```python
from build123d import *

# Parameters (mm, degrees)
SKETCH1_R           = 2.25
SKETCH1_R_2         = 1.5
BOSS_EXTRUDE1_DEPTH = 3


with BuildPart() as part:
    # Sketch1 → Boss-Extrude1 (new body)
    with BuildSketch(Plane.XY):
        with BuildLine():
            Line((-43.5, -20.5), (-47.6, -20.5))
            ThreePointArc((-47.6, -20.5), (-49.014213562, -19.914213562), (-49.6, -18.5))
            Line((-49.6, -18.5), (-49.6, 5))
            ThreePointArc((-49.6, 5), (-49.468344718, 5.71364418), (-49.090711985, 6.333333333))
            ThreePointArc((-49.090711985, 6.333333333), (-48.836067978, 7), (-49.090711985, 7.666666667))
            ThreePointArc((-49.090711985, 7.666666667), (-49.468344718, 8.28635582), (-49.6, 9))
            Line((-49.6, 9), (-49.6, 35))
            ThreePointArc((-49.6, 35), (-49.468344718, 35.71364418), (-49.090711985, 36.333333333))
            ThreePointArc((-49.090711985, 36.333333333), (-48.836067978, 37), (-49.090711985, 37.666666667))
            ThreePointArc((-49.090711985, 37.666666667), (-49.468344718, 38.28635582), (-49.6, 39))
            Line((-49.6, 39), (-49.6, 62.5))
            ThreePointArc((-49.6, 62.5), (-49.014213562, 63.914213562), (-47.6, 64.5))
            Line((-47.6, 64.5), (6.1, 64.5))
            ThreePointArc((6.1, 64.5), (7.514213562, 63.914213562), (8.1, 62.5))
            Line((8.1, 62.5), (8.1, 39))
            ThreePointArc((8.1, 39), (7.968344718, 38.28635582), (7.590711985, 37.666666667))
            ThreePointArc((7.590711985, 37.666666667), (7.336067978, 37), (7.590711985, 36.333333333))
            ThreePointArc((7.590711985, 36.333333333), (7.968344718, 35.71364418), (8.1, 35))
            Line((8.1, 35), (8.1, 9))
            ThreePointArc((8.1, 9), (7.968344718, 8.28635582), (7.590711985, 7.666666667))
            ThreePointArc((7.590711985, 7.666666667), (7.336067978, 7), (7.590711985, 6.333333333))
            ThreePointArc((7.590711985, 6.333333333), (7.968344718, 5.71364418), (8.1, 5))
            Line((8.1, 5), (8.1, -18.5))
            ThreePointArc((8.1, -18.5), (7.514213562, -19.914213562), (6.1, -20.5))
            Line((6.1, -20.5), (2, -20.5))
            ThreePointArc((2, -20.5), (0.585786438, -19.914213562), (0, -18.5))
            Line((0, -18.5), (0, 0))
            Line((0, 0), (-41.5, 0))
            Line((-41.5, 0), (-41.5, -18.5))
            ThreePointArc((-41.5, -18.5), (-42.085786438, -19.914213562), (-43.5, -20.5))
        make_face()
        with Locations((-45.55, -5.5)):
            Circle(SKETCH1_R, mode=Mode.SUBTRACT)
        with Locations((-45.55, -15)):
            Circle(SKETCH1_R, mode=Mode.SUBTRACT)
        with Locations((4.05, -5.5)):
            Circle(SKETCH1_R, mode=Mode.SUBTRACT)
        with Locations((4.05, -15)):
            Circle(SKETCH1_R, mode=Mode.SUBTRACT)
        with Locations((-30.55, 17)):
            Circle(SKETCH1_R, mode=Mode.SUBTRACT)
        with Locations((-30.55, 27)):
            Circle(SKETCH1_R, mode=Mode.SUBTRACT)
        with Locations((-10.14, 54.25)):
            Circle(SKETCH1_R_2, mode=Mode.SUBTRACT)
    extrude(amount=BOSS_EXTRUDE1_DEPTH)


solid = part.part
```
Can you work these out from the model? Positions are in its coordinate system, mm. A direction names the side the tool comes from. Round coordinates to 2 decimals unless told otherwise and drop trailing zeros. Loops run counter-clockwise (first coordinate to the right, second up) from the corner with the lowest first, then second, coordinate; pieces in that order, holes last.
Item 1: Will these pins go through, and if not, where does the flat tip stop? pin 1 Ø5 at (x, y) = (-30.55, 17) entering from -Z; pin 2 Ø0.9 at (x, z) = (-16.5, 1.5) entering from -Y.
Item 2: Please list where these lines run through material, in increasing order: L1, parallel to Y at x = 4.05, z = 2.2; L2, parallel to Y at x = -30.55, z = 1.35; L3, parallel to X at y = -10, z = 2.4.
Item 3: Suppose I cut it at B-B, the plane x = -30.55. Write out the boundary of the cut face in (y, z), then the cut area to 4 significant figures.
Item 4: Which directions (+Z, -Z, +X, -X, +Y, -Y) give clear straight access to the entire face, cutting with the end or side of a thin tool? Please do faces 1 (the flat face through (-20, 0, 1)), 2 (the flat face through (-49.6, -7, 1)).
Item 5: Suppose I cut it at A-A, the plane y = 17. Write out the boundary of the cut face in (x, z), then the cut area to 3 significant figures.
Item 6: If we mould it in two halves opening along Y, with no side actions, what happens to faces 3 (the flat face through (-20, 32, 3)), 4 (the cylindrical face through (7.5, 63.93, 1.48)), 5 (the cylindrical face through (-47.798, -5.401, 1.479))? For each: +Y half, -Y half, draft (parallel to the pull), parting line (faces both ways), or undercut.
Item 7: Suppose I cut it at C-C, the plane x = -10.14. Write out the boundary of the cut face in (y, z).
Item 8: Suppose I cut it at D-D, the plane z = 2.15. State how many separate pieces and enclosed holes the cut face has, then the cut area to 3 significant figures.
Reported:
1. pin 1: stops at z = 0
1. pin 2: stops at y = 0
2. L1: y = -20.5 to -17.25, -12.75 to -7.75, -3.25 to 64.5
2. L2: y = 0 to 14.75, 19.25 to 24.75, 29.25 to 64.5
2. L3: x = -49.6 to -41.5, 0 to 8.1
3. outline: (0, 0) - (14.75, 0) - (14.75, 3) - (0, 3) - close; (19.25, 0) - (24.75, 0) - (24.75, 3) - (19.25, 3) - close; (29.25, 0) - (64.5, 0) - (64.5, 3) - (29.25, 3) - close
3. area: 166.5 mm2
4. face 1: +Z, -Z, -Y
4. face 2: +Z, -Z, -X, +Y, -Y
5. outline: (-49.6, 0) - (-32.8, 0) - (-32.8, 3) - (-49.6, 3) - close; (-28.3, 0) - (8.1, 0) - (8.1, 3) - (-28.3, 3) - close
5. area: 160 mm2
6. face 3: draft
6. face 4: +Y half
6. face 5: undercut
7. outline: (0, 0) - (52.75, 0) - (52.75, 3) - (0, 3) - close; (55.75, 0) - (64.5, 0) - (64.5, 3) - (55.75, 3) - close
8. separate pieces: 1
8. enclosed holes: 7
8. area: 3,940 mm2
